The listing builds one solid part. Answer for the finished solid, in the listing's coordinates (mm). A direction names the side the tool comes from. Round coordinates to 2 decimals unless told otherwise and drop trailing zeros. Write each loop counter-clockwise with the first axis right and the second up, starting at its lowest first coordinate (ties: lowest second). Pieces come first, ordered by that corner, then holes.
(1) For faces 1 (the face through (-2, 18, 12.7)), 2 (the face through (0, 9.652, 8)), determine the directions among +Z, -Z, +X, -X, +Y, -Y from which every point of the face is accessible in a straight line to the end or side of a thin tool.
(2) A cutting plane is placed at C-C, the plane x = -119. Give the vertices of the cut face in (y, z).
(3) A cutting plane is placed at D-D, the plane x = -39.5. Give the vertices of the cut face in (y, z).
(4) A cutting plane is placed at A-A, the plane z = 10.5. Give the vertices of the cut face in (x, y).
(5) Find the intervals of material crossed by probe 1 along X at (y, z) = (-51, 9.75); probe 2 along X at (y, z) = (-5.5, 4.25); probe 3 along Y at (x, z) = (85.5, 7.5), in increasing order.
(6) Each of these flat-tipped pins is pushed along its axis until it touches: pin 1 Ø4 at (y, z) = (15.5, 6.5) entering from -X; pin 2 Ø4.5 at (x, z) = (-3, 9) entering from +Y; pin 3 Ø3 at (y, z) = (30, 2.5) entering from +X. Where does it stop, or does it pass through?
(7) A cutting plane is placed at B-B, the plane y = 37. Give the vertices of the cut face in (x, z), and give its area (3 significant figures).
(8) The mould has two halves that part along Y. Classify faces 3 (the face through (-4.4, 2.3, 3.81)), 4 (the face through (-2.03, -25.41, 6.26)), 5 (the face through (-152.396, 1.117, 6.261)): +Y half, -Y half, draft (parallel to the pull), parting line (faces both ways), or undercut.
from build123d import *

# Parameters (mm, degrees)
F1_DEPTH = 12.7
F2_R     = 4.6355
F3_DEPTH = 12.7
F4_W     = 19.304
F4_H     = 19.304
F4_R     = 4.6355
F5_DEPTH = 8.89


with BuildPart() as f1:
    # F0 (on Top) → F1 (new body)
    with BuildSketch(Plane.XY):
        with BuildLine():
            ThreePointArc((131.9822715367, -76.2), (147.2070959265, -39.4440224736), (152.4, 0))
            ThreePointArc((152.4, 0), (147.2070959265, 39.4440224736), (131.9822715368, 76.2))
            ThreePointArc((131.9822715367, 76.2), (70.7106074079, 38.5384530031), (0, 25.4))
            ThreePointArc((0, 25.4), (-70.7106074079, 38.5384530031), (-131.9822715367, 76.2))
            ThreePointArc((-131.9822715368, 76.2), (-152.4, 0), (-131.9822715367, -76.2))
            ThreePointArc((-131.9822715367, -76.2), (0, -25.4), (131.9822715367, -76.2))
        make_face()
    extrude(amount=F1_DEPTH)

    # F2 (on face) → F3 (cut, through all)
    with BuildSketch(Plane.XY.offset(12.7)):
        Circle(F2_R)
    extrude(amount=-F3_DEPTH, mode=Mode.SUBTRACT)

    # F4 (on face) → F5 (cut)
    with BuildSketch(Plane.XY.offset(12.7)):
        Rectangle(F4_W, F4_H)
        Circle(F4_R, mode=Mode.SUBTRACT)
    extrude(amount=-F5_DEPTH, mode=Mode.SUBTRACT)


solid = f1.part
Solutions:
1. face 1: +Z, +X, -X, +Y, -Y
1. face 2: +Z
2. outline: (-65.44, 0) - (65.44, 0) - (65.44, 12.7) - (-65.44, 12.7) - close
3. outline: (-29.4, 0) - (29.4, 0) - (29.4, 12.7) - (-29.4, 12.7) - close
4. outline: (-131.98, -76.2) arc R196.85 cw to (131.98, -76.2) arc R152.4 ccw to (131.98, 76.2) arc R196.85 cw to (-131.98, 76.2) arc R152.4 ccw to start; hole (-9.65, -9.65) - (9.65, -9.65) - (9.65, 9.65) - (-9.65, 9.65) - close
5. probe 1: x = -143.61 to -97.07, 97.07 to 143.61
5. probe 2: x = -152.3 to -9.65, 9.65 to 152.3
5. probe 3: y = -44.94 to 44.94
6. pin 1: stops at x = -151.8
6. pin 2: stops at y = 25.47
6. pin 3: stops at x = 149.71
7. outline: (-147.84, 0) - (-66.58, 0) - (-66.58, 12.7) - (-147.84, 12.7) - close; (66.58, 0) - (147.84, 0) - (147.84, 12.7) - (66.58, 12.7) - close
7. area: 2,060 mm2
8. face 3: undercut
8. face 4: -Y half
8. face 5: parting line
